Build history of the part. All positions in model axes, mm. Face numbers are marked on the shaded views. A direction names the side the tool comes from. Coordinates: 2 decimals unless noted, no trailing zeros. Order: outer loops, then holes, each group sorted by start corner. A loop starts at its lowest first (then second) coordinate and runs counter-clockwise, first axis right, second up. Notation, with made-up numbers: (-17, 51.5) - (21, 51.5) arc R20 ccw to (21, 58.5) - close; hole circle Ø1 at (4.25, 36.25). An arc over 180 degrees is marked (long way). Return JSON: item names as keys, results as strings.
from build123d import *

# Parameters (mm, degrees)
PAD_DEPTH            = 46
PAD_DEPTH_BACK       = 30
SKETCH009_R          = 8.650139
POCKET006_DEPTH      = 4.25
SKETCH011_R          = 1.5
POCKET008_DEPTH      = 9.501
POCKET008_DEPTH_BACK = 0.001
SKETCH010_R          = 8.650139
SKETCH010_R_2        = 3
POCKET007_DEPTH      = 5
SKETCH005_R          = 5.8
POCKET002_DEPTH      = 9.501
POCKET002_DEPTH_BACK = 0.001
SKETCH006_R          = 6.1
POCKET003_DEPTH      = 5.75
POCKET004_DEPTH      = 9.501
POCKET004_DEPTH_BACK = 0.001
SKETCH008_W          = 4
SKETCH008_H          = 12.2
POCKET005_DEPTH      = 5.75
POCKET009_DEPTH      = 9.501
POCKET009_DEPTH_BACK = 0.001
POCKET_DEPTH         = 2.751
SKETCH014_R          = 3.035
POCKET010_DEPTH      = 31.001
PAD001_DEPTH         = 9.5
SKETCH017_R          = 1.6
POCKET011_DEPTH      = 9.501
SKETCH018_W          = 100
SKETCH018_H          = 100
POCKET012_DEPTH      = 5.501
SKETCH020_R          = 8
SKETCH019_R          = 6
SKETCH021_R          = 8
POCKET013_DEPTH      = 5.501
SKETCH023_W          = 100
SKETCH023_H          = 16
SKETCH022_W          = 100
SKETCH022_H          = 12
SKETCH024_W          = 100
SKETCH024_H          = 16
SKETCH025_R          = 1.6
POCKET014_DEPTH      = 9.501
POCKET015_DEPTH      = 3
FILLET_R             = 3
FILLET001_R          = 2
FILLET002_R          = 0.43
FILLET003_R          = 3
SKETCH027_W          = 50
SKETCH027_H          = 0.5
POCKET016_DEPTH      = 4.25


with BuildPart() as part:
    # Sketch → Pad (new body, two sides)
    with BuildSketch(Plane.YZ) as pad_sk:
        Polygon((0, -9.5), (22, -9.5), (22, 0), (-22, 0), (-22, -9.5), align=None)
    extrude(amount=PAD_DEPTH)
    extrude(pad_sk.sketch, amount=-PAD_DEPTH_BACK)

    # Sketch009 → Pocket006 (cut, symmetric)
    with BuildSketch(Plane.XY):
        with Locations((5, -17.25)):
            Circle(SKETCH009_R)
        with Locations((5, 17.25)):
            Circle(SKETCH009_R)
    extrude(amount=POCKET006_DEPTH, both=True, mode=Mode.SUBTRACT)

    # Sketch011 → Pocket008 (cut, two sides)
    with BuildSketch(Plane.XY) as pocket008_sk:
        with Locations((5, 17.25)):
            Circle(SKETCH011_R)
        with Locations((5, -17.25)):
            Circle(SKETCH011_R)
    extrude(amount=-POCKET008_DEPTH, mode=Mode.SUBTRACT)
    extrude(pocket008_sk.sketch, amount=POCKET008_DEPTH_BACK, mode=Mode.SUBTRACT)

    # Sketch010 → Pocket007 (cut, symmetric)
    with BuildSketch(Plane.XY):
        with Locations((5, -17.25)):
            Circle(SKETCH010_R)
        with Locations((5, -17.25)):
            Circle(SKETCH010_R_2, mode=Mode.SUBTRACT)
        with Locations((5, 17.25)):
            Circle(SKETCH010_R)
        with Locations((5, 17.25)):
            Circle(SKETCH010_R_2, mode=Mode.SUBTRACT)
    extrude(amount=POCKET007_DEPTH, both=True, mode=Mode.SUBTRACT)

    # Sketch005 → Pocket002 (cut, two sides)
    with BuildSketch(Plane.XY) as pocket002_sk:
        with Locations((9, 0)):
            Circle(SKETCH005_R)
    extrude(amount=-POCKET002_DEPTH, mode=Mode.SUBTRACT)
    extrude(pocket002_sk.sketch, amount=POCKET002_DEPTH_BACK, mode=Mode.SUBTRACT)

    # Sketch006 → Pocket003 (cut)
    with BuildSketch(Plane.XY):
        with Locations((9, 0)):
            Circle(SKETCH006_R)
    extrude(amount=-POCKET003_DEPTH, mode=Mode.SUBTRACT)

    # Sketch007 → Pocket004 (cut, two sides)
    with BuildSketch(Plane.XY) as pocket004_sk:
        Polygon((9, 0), (11.086323, 5.732125), (11.220218, 6.1), (111.220218, 6.1), (111.220218, -6.1), (11.220218, -6.1), (11.086323, -5.732125), align=None)
    extrude(amount=-POCKET004_DEPTH, mode=Mode.SUBTRACT)
    extrude(pocket004_sk.sketch, amount=POCKET004_DEPTH_BACK, mode=Mode.SUBTRACT)

    # Sketch008 → Pocket005 (cut)
    with BuildSketch(Plane.XY):
        with Locations((11, 0)):
            Rectangle(SKETCH008_W, SKETCH008_H)
    extrude(amount=-POCKET005_DEPTH, mode=Mode.SUBTRACT)

    # Sketch012 → Pocket009 (cut, two sides)
    with BuildSketch(Plane.XY) as pocket009_sk:
        with BuildLine():
            ThreePointArc((31.8, 12.35), (30.2, 10.75), (31.8, 9.15))
            Line((31.8, 9.15), (36.2, 9.15))
            ThreePointArc((36.2, 9.15), (37.8, 10.75), (36.2, 12.35))
            Line((31.8, 12.35), (36.2, 12.35))
        make_face()
        with BuildLine():
            ThreePointArc((31.8, -9.15), (30.2, -10.75), (31.8, -12.35))
            Line((31.8, -12.35), (36.2, -12.35))
            ThreePointArc((36.2, -12.35), (37.8, -10.75), (36.2, -9.15))
            Line((31.8, -9.15), (36.2, -9.15))
        make_face()
    extrude(amount=-POCKET009_DEPTH, mode=Mode.SUBTRACT)
    extrude(pocket009_sk.sketch, amount=POCKET009_DEPTH_BACK, mode=Mode.SUBTRACT)

    # Sketch013 (on DatumPlane) → Pocket (cut, through all)
    with BuildSketch(Plane.XY.offset(-6.75)):
        with BuildLine():
            ThreePointArc((9, 6.1), (2.9, 0), (9, -6.1))
            Line((9, -6.1), (34, -6.1))
            Line((34, 6.1), (34, -6.1))
            Line((9, 6.1), (34, 6.1))
        make_face()
    extrude(amount=-POCKET_DEPTH, mode=Mode.SUBTRACT)

    # Sketch014 (on DatumPlane) → Pocket010 (cut, through all)
    with BuildSketch(Plane.YZ.offset(15)):
        with Locations((-16, 0)):
            Circle(SKETCH014_R)
        with Locations((16, 0)):
            Circle(SKETCH014_R)
    extrude(amount=POCKET010_DEPTH, mode=Mode.SUBTRACT)

    # Sketch016 → Pad001 (join)
    with BuildSketch(Plane.XY):
        Polygon((13, -22), (46, -22), (46, -24), (15.856296, -24), align=None)
        Polygon((13, 22), (46, 22), (46, 24), (15.856296, 24), align=None)
    extrude(amount=-PAD001_DEPTH)

    # Sketch017 → Pocket011 (cut, through all)
    with BuildSketch(Plane.XY):
        with Locations((26.25, -10.75)):
            Circle(SKETCH017_R)
        with Locations((26.25, -21.25)):
            Circle(SKETCH017_R)
        with Locations((41.75, -21.25)):
            Circle(SKETCH017_R)
        with Locations((41.75, -10.75)):
            Circle(SKETCH017_R)
        with Locations((26.25, 10.75)):
            Circle(SKETCH017_R)
        with Locations((41.75, 10.75)):
            Circle(SKETCH017_R)
        with Locations((26.25, 21.25)):
            Circle(SKETCH017_R)
        with Locations((41.75, 21.25)):
            Circle(SKETCH017_R)
        with Locations((17, -10)):
            Circle(SKETCH017_R)
        with Locations((17, 10)):
            Circle(SKETCH017_R)
        with Locations((2, -6)):
            Circle(SKETCH017_R)
        with Locations((2, 6)):
            Circle(SKETCH017_R)
    extrude(amount=-POCKET011_DEPTH, mode=Mode.SUBTRACT)

    # Sketch018 (on DatumPlane) → Pocket012 (cut, through all)
    with BuildSketch(Plane.XY.offset(-5.5)):
        with Locations((-51.1, 0)):
            Rectangle(SKETCH018_W, SKETCH018_H)
    extrude(amount=POCKET012_DEPTH, mode=Mode.SUBTRACT)

    # Sketch020 (on DatumPlane) → SubtractiveLoft section 0
    with BuildSketch(Plane.XY.offset(-5.5)):
        with Locations((-7, 0)):
            Circle(SKETCH020_R)
    # Sketch019 (on DatumPlane) → SubtractiveLoft section 1
    with BuildSketch(Plane.XY.offset(-7.5)):
        with Locations((-7, 0)):
            Circle(SKETCH019_R)
    # Sketch021 (on DatumPlane) → SubtractiveLoft section 2
    with BuildSketch(Plane.XY.offset(-9.5)):
        with Locations((-7, 0)):
            Circle(SKETCH021_R)
    loft(ruled=True, mode=Mode.SUBTRACT)

    # Sketch020 (on DatumPlane) → Pocket013 (cut, through all)
    with BuildSketch(Plane.XY.offset(-5.5)):
        with Locations((-7, 0)):
            Circle(SKETCH020_R)
    extrude(amount=POCKET013_DEPTH, mode=Mode.SUBTRACT)

    # Sketch023 (on DatumPlane) → SubtractiveLoft001 section 0
    with BuildSketch(Plane.XY.offset(-5.5)):
        with Locations((-57, 0)):
            Rectangle(SKETCH023_W, SKETCH023_H)
    # Sketch022 (on DatumPlane) → SubtractiveLoft001 section 1
    with BuildSketch(Plane.XY.offset(-7.5)):
        with Locations((-57, 0)):
            Rectangle(SKETCH022_W, SKETCH022_H)
    # Sketch024 (on DatumPlane) → SubtractiveLoft001 section 2
    with BuildSketch(Plane.XY.offset(-9.5)):
        with Locations((-57, 0)):
            Rectangle(SKETCH024_W, SKETCH024_H)
    loft(ruled=True, mode=Mode.SUBTRACT)

    # Sketch025 → Pocket014 (cut, through all)
    with BuildSketch(Plane.XY):
        with Locations((-24, -14)):
            Circle(SKETCH025_R)
        with Locations((-24, 14)):
            Circle(SKETCH025_R)
    extrude(amount=-POCKET014_DEPTH, mode=Mode.SUBTRACT)

    # Sketch026 (on DatumPlane) → Pocket015 (cut)
    with BuildSketch(Plane.XY.offset(-9.5)):
        Polygon((26.25, 24.569764), (23.375, 22.909882), (23.375, 19.590118), (26.25, 17.930236), (29.125, 19.590118), (29.125, 22.909882), align=None)
        Polygon((44.625, 22.909882), (41.75, 24.569764), (38.875, 22.909882), (38.875, 19.590118), (41.75, 17.930236), (44.625, 19.590118), align=None)
        Polygon((44.625, 9.090118), (44.625, 12.409882), (41.75, 14.069764), (38.875, 12.409882), (38.875, 9.090118), (41.75, 7.430236), align=None)
        Polygon((29.125, 9.090118), (29.125, 12.409882), (26.25, 14.069764), (23.375, 12.409882), (23.375, 9.090118), (26.25, 7.430236), align=None)
        Polygon((29.125, -12.409882), (29.125, -9.090118), (26.25, -7.430236), (23.375, -9.090118), (23.375, -12.409882), (26.25, -14.069764), align=None)
        Polygon((41.75, -14.069764), (44.625, -12.409882), (44.625, -9.090118), (41.75, -7.430236), (38.875, -9.090118), (38.875, -12.409882), align=None)
        Polygon((44.625, -22.909882), (44.625, -19.590118), (41.75, -17.930236), (38.875, -19.590118), (38.875, -22.909882), (41.75, -24.569764), align=None)
        Polygon((29.125, -19.590118), (26.25, -17.930236), (23.375, -19.590118), (23.375, -22.909882), (26.25, -24.569764), (29.125, -22.909882), align=None)
    extrude(amount=POCKET015_DEPTH, mode=Mode.SUBTRACT)

    # Fillet
    fillet_edges = [part.edges().sort_by_distance(p)[0] for p in [
        (-30, -22, -7.5),
        (-30, 22, -7.5),
        (-30, 7, -6.5),
        (-30, 7, -8.5),
        (-30, -7, -6.5),
        (-30, -7, -8.5),
    ]]
    fillet(fillet_edges, radius=FILLET_R)

    # Fillet001
    fillet001_edges = [part.edges().sort_by_distance(p)[0] for p in [
        (-1.1, -11.1169, -2.125),
        (-1.1, 11.1169, -2.125),
    ]]
    fillet(fillet001_edges, radius=FILLET001_R)

    # Fillet002
    fillet002_edges = [part.edges().sort_by_distance(p)[0] for p in [
        (12.229275, -22, -2.125),
        (12.229275, 22, -2.125),
    ]]
    fillet(fillet002_edges, radius=FILLET002_R)

    # Fillet003
    fillet003_edges = [part.edges().sort_by_distance(p)[0] for p in [
        (-1.1, -22, -5.25),
        (-1.1, 22, -5.25),
    ]]
    fillet(fillet003_edges, radius=FILLET003_R)

    # Sketch027 → Pocket016 (cut, symmetric)
    with BuildSketch(Plane.XY):
        with Locations((21, -23.75)):
            Rectangle(SKETCH027_W, SKETCH027_H)
        with Locations((21, 23.75)):
            Rectangle(SKETCH027_W, SKETCH027_H)
    extrude(amount=POCKET016_DEPTH, both=True, mode=Mode.SUBTRACT)


solid = part.part
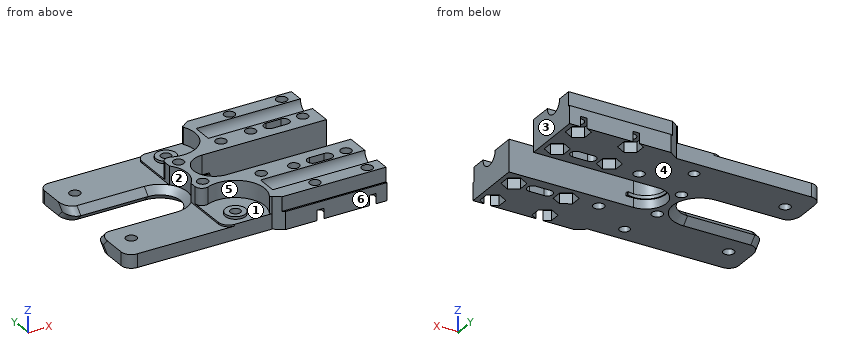
1. Drop flat-ended pins along their axis: pin 1 (2 mm diameter, centred on y = 2, z = -7, fed in from -X); pin 2 (1.7 mm diameter, centred on x = 26.5, y = -11.5, fed in from -Z); pin 3 (3 mm diameter, centred on y = 13.5, z = -1.5, fed in from -X). Give the stop position or say it passes through.
Check values:
{"pin 1": "x = -1.73", "pin 2": "z = -6.5", "pin 3": "x = 11.87"}
2. Cut at A-A on x = 17. Give the cut face in (y, z) (3 decimals), plus the area to 3 significant figures.
Check values:
{"outline": "(-24, -9.5) - (-11.6, -9.5) - (-11.6, 0) - (-12.965, 0) arc R3.035 cw to (-19.035, 0) - (-23.5, 0) - (-23.5, -4.25) - (-24, -4.25) - close; (-8.4, -9.5) - (-6.1, -9.5) - (-6.1, 0) - (-8.4, 0) - close; (6.1, -9.5) - (8.4, -9.5) - (8.4, 0) - (6.1, 0) - close; (11.6, -9.5) - (24, -9.5) - (24, -4.25) - (23.5, -4.25) - (23.5, 0) - (19.035, 0) arc R3.035 cw to (12.965, 0) - (11.6, 0) - close", "area": "246 mm²"}
3. Cut at B-B on x = 31. Give the cut face in (y, z) (3 decimals), plus the area to 3 significant figures.
Check values:
{"outline": "(-24, -9.5) - (-12.136, -9.5) - (-12.136, 0) - (-12.965, 0) arc R3.035 cw to (-19.035, 0) - (-23.5, 0) - (-23.5, -4.25) - (-24, -4.25) - close; (-9.364, -9.5) - (-6.1, -9.5) - (-6.1, 0) - (-9.364, 0) - close; (6.1, -9.5) - (9.364, -9.5) - (9.364, 0) - (6.1, 0) - close; (12.136, -9.5) - (24, -9.5) - (24, -4.25) - (23.5, -4.25) - (23.5, 0) - (19.035, 0) arc R3.035 cw to (12.965, 0) - (12.136, 0) - close", "area": "254 mm²"}
4. Cut at C-C on x = 5. State how many separate pieces and enclosed holes the cut face has, plus the area to 3 significant figures.
Check values:
{"separate pieces": "4", "enclosed holes": "0", "area": "175 mm²"}
5. Probe L1, parallel to Y at x = 5, z = -5.65; L2, parallel to Y at x = -14, z = -7.5; L3, parallel to Y at x = 29, z = -2.5. List the from-to ranges inside material, lowest first.
Check values:
{"L1": "-22 to -18.75, -15.75 to -4.61, 4.61 to 15.75, 18.75 to 22", "L2": "-22 to -6, 6 to 22", "L3": "-23.5 to -17.72, -14.28 to -6.1, 6.1 to 14.28, 17.72 to 23.5"}
6. Tool access for the marked faces 1, 2 and 3: list every direction of +Z, -Z, +X, -X, +Y, -Y with a clear straight run to the whole face (end or side of a thin tool).
Check values:
{"face 1": "+Z", "face 2": "+Z, -X", "face 3": "+Z, -Z, +X, +Y, -Y"}
7. Mould opens along Y. For the marked faces 4, 5 and 6 say: pulls with the +Y half, pulls with the -Y half, needs draft (parallel to the pull), parting line crosses it, or undercut.
Check values:
{"face 4": "needs draft", "face 5": "undercut", "face 6": "pulls with the -Y half"}
